Geometry check sheet. Reference: the model listing, model coordinates, mm. Face numbers are marked on the shaded views. A direction names the side the tool comes from. Round coordinates to 2 decimals unless told otherwise and drop trailing zeros. Write each loop counter-clockwise with the first axis right and the second up, starting at its lowest first coordinate (ties: lowest second). Pieces come first, ordered by that corner, then holes.
from build123d import *

# Parameters (mm, degrees)
PAD_DEPTH       = 156
SKETCH001_W     = 31
SKETCH001_H     = 25
POCKET_DEPTH    = 20.001
SKETCH002_W     = 170
SKETCH002_H     = 36
POCKET001_DEPTH = 4
SKETCH003_W     = 140
SKETCH003_H     = 140
POCKET002_DEPTH = 12
SKETCH004_W     = 170
SKETCH004_H     = 40
PAD001_DEPTH    = 8
FILLET_R        = 1
CHAMFER_SIZE    = 3
CHAMFER001_SIZE = 1
CHAMFER002_SIZE = 3
CHAMFER003_SIZE = 11.8


with BuildPart() as part:
    # Sketch → Pad (new body)
    with BuildSketch(Plane.XZ):
        Polygon((-80, 20), (-80, 5), (-85, 5), (-85, 0), (85, 0), (85, 5), (80, 5), (80, 20), align=None)
    extrude(amount=-PAD_DEPTH)

    # Sketch001 (on Face2 of Pad) → Pocket (cut, through all)
    with BuildSketch(Plane.XY.offset(20)):
        with Locations((0, 85)):
            Rectangle(SKETCH001_W, SKETCH001_H)
    extrude(amount=-POCKET_DEPTH, mode=Mode.SUBTRACT)

    # Sketch002 (on Face14 of Pocket) → Pocket001 (cut)
    with BuildSketch(Plane(origin=(0, 0, 0), x_dir=(1, 0, 0), z_dir=(0, 0, -1))):
        with Locations((0, -85)):
            Rectangle(SKETCH002_W, SKETCH002_H)
    extrude(amount=-POCKET001_DEPTH, mode=Mode.SUBTRACT)

    # Sketch003 (on Face3 of Pocket001) → Pocket002 (cut)
    with BuildSketch(Plane.XY.offset(20)):
        with Locations((0, 78)):
            Rectangle(SKETCH003_W, SKETCH003_H)
    extrude(amount=-POCKET002_DEPTH, mode=Mode.SUBTRACT)

    # Sketch004 (on Face4 of Pocket002) → Pad001 (join)
    with BuildSketch(Plane.XZ):
        with Locations((0, 20)):
            Rectangle(SKETCH004_W, SKETCH004_H)
    extrude(amount=PAD001_DEPTH)

    # Fillet
    fillet_edges = [part.edges().sort_by_distance(p)[0] for p in [
        (0, 72.5, 8),
        (-15.5, 85, 8),
        (0, 97.5, 8),
        (15.5, 85, 8),
    ]]
    fillet(fillet_edges, radius=FILLET_R)

    # Chamfer
    chamfer_edges = [part.edges().sort_by_distance(p)[0] for p in [
        (-80, 78, 20),
        (0, 156, 20),
        (80, 78, 20),
    ]]
    chamfer(chamfer_edges, length=CHAMFER_SIZE)

    # Chamfer001
    chamfer001_edges = [part.edges().sort_by_distance(p)[0] for p in [
        (0, 67, 0),
        (0, 103, 0),
    ]]
    chamfer(chamfer001_edges, length=CHAMFER001_SIZE)

    # Chamfer002
    chamfer002_edges = [part.edges().sort_by_distance(p)[0] for p in [
        (0, 0, 40),
        (85, -4, 40),
        (0, -8, 40),
        (-85, -4, 40),
    ]]
    chamfer(chamfer002_edges, length=CHAMFER002_SIZE)

    # Chamfer003
    chamfer003_edges = [part.edges().sort_by_distance(p)[0] for p in [
        (0, 148, 8),
        (-70, 78, 8),
        (70, 78, 8),
        (0, 8, 8),
    ]]
    chamfer(chamfer003_edges, length=CHAMFER003_SIZE)


solid = part.part
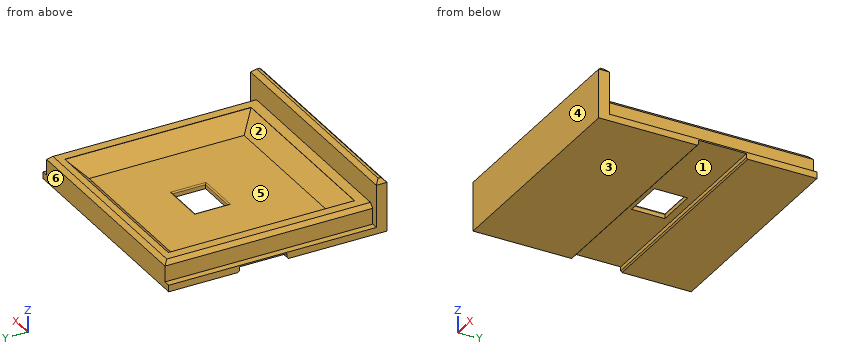
1. Section check B-B (x = -9.5). Record the cut outline in (y, z), plus the area to 3 significant figures.
2. Access from +Z, -Z, +X, -X, +Y, -Y to the whole of each face (thin tool, end or side, straight path). Record for the marked faces 1, 2 and 3.
3. Scan lines: line 1 along Z through (x, y) = (48, 95); line 2 along Y through (x, z) = (-68, 28); line 3 along Y through (x, z) = (-27, 19). Record each from-to range of solid material in increasing order.
4. Section check A-A (z = 10). Record the cut outline in (x, y), plus the area to 3 significant figures.
5. Section check C-C (y = 77.5). Record the cut outline in (x, z).
6. Release check for a two-part mould opening along Y. For the marked faces 4, 5 and 6 record: +Y half, -Y half, draft (parallel to the pull), parting line (faces both ways), or undercut.
7. Depth check by flat-ended pin: pin 1 Ø1.5 at (x, y) = (58.5, 101.5) entering from -Z; pin 2 Ø5.5 at (x, y) = (82.5, 81) entering from +Z; pin 3 Ø8 at (x, z) = (-14, 25.5) entering from +Y. Enter the tip coordinate at first touch or a pass-through.
8. Section check D-D (x = -44.5). Record the cut outline in (y, z), plus the area to 3 significant figures.
Results below:
1. outline: (-8, 0) - (66, 0) - (67, 1) - (67, 4) - (72.5, 4) - (72.5, 7) arc R1 ccw to (71.5, 8) - (19.8, 8) - (8, 19.8) - (8, 20) - (0, 20) - (0, 37) - (-3, 40) - (-5, 40) - (-8, 37) - close; (97.5, 4) - (103, 4) - (103, 1) - (104, 0) - (156, 0) - (156, 17) - (153, 20) - (148, 20) - (148, 19.8) - (136.2, 8) - (98.5, 8) arc R1 ccw to (97.5, 7) - close
1. area: 1,640 mm2
2. face 1: -Z, +X, -X
2. face 2: +Z
2. face 3: -Z, +X, -X, +Y, -Y
3. line 1: z = 4 to 8
3. line 2: y = -8 to 0
3. line 3: y = -8 to 8.8, 147.2 to 154
4. outline: (-85, -8) - (85, -8) - (85, 0) - (80, 0) - (80, 156) - (-80, 156) - (-80, 0) - (-85, 0) - close; hole (-60.2, 17.8) - (60.2, 17.8) - (60.2, 138.2) - (-60.2, 138.2) - close
4. area: 11,800 mm2
5. outline: (-85, 4) - (-15.5, 4) - (-15.5, 7) arc R1 ccw to (-16.5, 8) - (-58.2, 8) - (-70, 19.8) - (-70, 20) - (-77, 20) - (-80, 17) - (-80, 5) - (-85, 5) - close; (15.5, 4) - (85, 4) - (85, 5) - (80, 5) - (80, 17) - (77, 20) - (70, 20) - (70, 19.8) - (58.2, 8) - (16.5, 8) arc R1 ccw to (15.5, 7) - close
6. face 4: -Y half
6. face 5: undercut
6. face 6: +Y half
7. pin 1: stops at z = 4
7. pin 2: stops at z = 17.25
7. pin 3: stops at y = 0
8. outline: (-8, 0) - (66, 0) - (67, 1) - (67, 4) - (103, 4) - (103, 1) - (104, 0) - (156, 0) - (156, 17) - (153, 20) - (148, 20) - (148, 19.8) - (136.2, 8) - (19.8, 8) - (8, 19.8) - (8, 20) - (0, 20) - (0, 37) - (-3, 40) - (-5, 40) - (-8, 37) - close
8. area: 1,740 mm2
